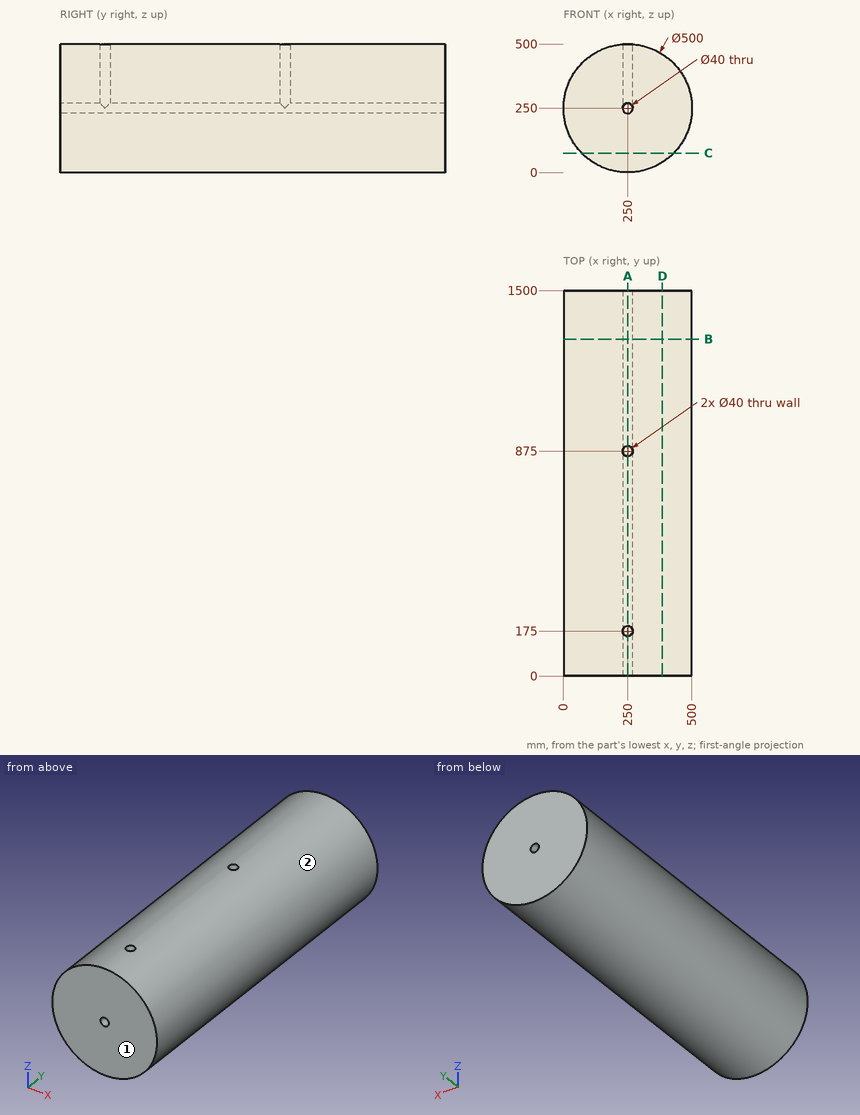
Design review of the part shown in the three views and the two pictorial views. Dimensions are in mm from the part's minimum x, y and z. Round coordinates to 2 decimals unless told otherwise and drop trailing zeros. Loops run counter-clockwise (first coordinate to the right, second up) from the corner with the lowest first, then second, coordinate; pieces in that order, holes last.
1) Wall thickness on line 1 along Y through (x, z) = (250, 443); line 2 along X through (y, z) = (69.5, 248.5); line 3 along X through (y, z) = (403, 241.5): over which ranges is each line inside the solid? List them lowest first.
Values follow:
line 1: y = 0 to 155, 195 to 855, 895 to 1500
line 2: x = 0 to 230.06, 269.94 to 500
line 3: x = 0.14 to 231.9, 268.1 to 499.86
2) Consider section A-A on x = 250. State the section outline as (y, z) points, then the cut area to 3 significant figures.
Values follow:
outline: (0, 0) - (1500, 0) - (1500, 230) - (0, 230) - close; (0, 270) - (155, 270) - (155, 500) - (0, 500) - close; (195, 270) - (855, 270) - (855, 500) - (195, 500) - close; (895, 270) - (1500, 270) - (1500, 500) - (895, 500) - close
area: 672,000 mm2
3) The part is to be moulded in two halves that separate along Z. For the marked faces 1 and 2, say which applies: pulls with the +Z half, pulls with the -Z half, needs draft (parallel to the pull), parting line crosses it, or undercut.
Values follow:
face 1: needs draft
face 2: parting line crosses it
4) Consider section B-B on y = 1310.5. State the section outline as (x, z) points, then the cut area to 3 significant figures.
Values follow:
outline: circle Ø500 at (250, 250); hole circle Ø40 at (250, 250)
area: 195,000 mm2
5) Clearance check with flat-ended pins moving along their axes: P1, Ø2, axis at y = 293, z = 400.5, coming from the +X side; P2, Ø1, axis at x = 315.5, y = 377.5, coming from the +Z side; P3, Ø1.5, axis at y = 1143.5, z = 161.5, coming from the -X side. State where each tip first meets the part, or that it passes through.
Values follow:
P1: stops at x = 450.37
P2: stops at z = 491.4
P3: stops at x = 15.91
6) Consider section D-D on x = 384.5. State the section outline as (y, z) points.
Values follow:
outline: (0, 39.26) - (1500, 39.26) - (1500, 460.74) - (0, 460.74) - close
7) Consider section C-C on z = 75.5. State the section outline as (x, y) points.
Values follow:
outline: (70.98, 0) - (429.02, 0) - (429.02, 1500) - (70.98, 1500) - close
